Autodesk Inventor part; units mm, degrees
ref_plane "YZ Plane" through (0, 0, 0) normal (1, 0, 0) x (0, 1, 0)
ref_plane "XZ Plane" through (0, 0, 0) normal (0, 1, 0) x (-1, 0, 0)
ref_plane "XY Plane" through (0, 0, 0) normal (0, 0, 1) x (1, 0, 0)
sketch "Sketch1" plane through (0, 0, 0) normal (0, 1, 0) x (-1, 0, 0)
  line L0 (15, 25) -> (-15, 25)
  line L1 (-15, 25) -> (-15, -25)
  line L2 (-15, -25) -> (15, -25)
  line L3 (15, -25) -> (15, 25)
  line L4 (21, 0) -> (-21, 0) construction
  line L5 (0, -35) -> (0, 35) construction
  point P0 (0, 0)
  dimension "d11" = 15
  dimension "d12" = 15
  dimension "d13" = 25
  dimension "d14" = 25
extrude "Extrusion1" add sketch "Sketch1" against normal blind 1
fillet "Fillet1" radius 2.5 2 edges at (-15, -0.5, 25) (15, -0.5, 25)
fillet "Fillet2" radius 4 2 edges at (-15, -0.5, -25) (15, -0.5, -25)
sketch "Sketch3" plane through (0, 0, 0) normal (0, 1, 0) x (1, 0, 0)
  arc A0 (15, 21) -> (11, 25) centre (11, 21) ccw
  arc A1 (-11, 25) -> (-15, 21) centre (-11, 21) ccw
  line L0 (15, -22.5) -> (15, 21)
  line L1 (-15, 21) -> (-15, -22.5)
  line L2 (-12.5, -25) -> (12.5, -25)
  point P0 (0, 0)
  point P1 (11, -7)
  point P2 (-11, -8.5)
  point P3 (12.5, -25)
  dimension "d24" = 4
  dimension "d25" = 4
  dimension "d52" = 18
  dimension "d53" = 1.5
hole "Hole2" at (-11, 0, -21) at (11, 0, -21) at (11, 0, 7) at (-11, 0, 8.5) direction (0, -1, 0) diameter 3.4 end through all
properties part number "mcu_pcb"
The listing builds one solid part. Answer for the finished solid, in the listing's coordinates (mm). Give positions to 0.01 mm unless a question says otherwise; leave off trailing zeros. Write each loop counter-clockwise with the first axis right and the second up, starting at its lowest first coordinate (ties: lowest second). Pieces come first, ordered by that corner, then holes. Notation, with made-up numbers: (72.25, 63) -> (78.25, 63) arc R11 ccw to (78.25, 76) -> close; hole circle Ø1 at (42, 52.5). An arc over 180 degrees is marked (long way). One line per question, with ' | ' between items. Start each with the question number.
1. Section A-A (y = -0.25) is taken. Determine the outline of the cut face in (x, z), plus the area to 3 significant figures.
2. Find the intervals of material crossed by probe 1 along X at (y, z) = (-0.6, -21); probe 2 along Z at (x, y) = (11, -0.25); probe 3 along Z at (x, y) = (-9.75, -0.55), in increasing order.
3. For a pull along X with two mould halves and no side action, classify faces 1 (the cylindrical face through (-13.859, -0.507, -23.797)), 2 (the cylindrical face through (12.66, -0.51, 6.63)), 3 (the cylindrical face through (14.287, -0.507, 24.248)) as pulls with the +X half, pulls with the -X half, needs draft (parallel to the pull), parting line crosses it, or undercut.
Response values:
1) outline: (-15, -21) arc R4 ccw to (-11, -25) -> (11, -25) arc R4 ccw to (15, -21) -> (15, 22.5) arc R2.5 ccw to (12.5, 25) -> (-12.5, 25) arc R2.5 ccw to (-15, 22.5) -> close; hole circle Ø3.4 at (-11, -21); hole circle Ø3.4 at (-11, 8.5); hole circle Ø3.4 at (11, -21); hole circle Ø3.4 at (11, 7) | area: 1,450 mm2
2) probe 1: -15 to -12.7, -9.3 to 9.3, 12.7 to 15 | probe 2: -25 to -22.7, -19.3 to 5.3, 8.7 to 25 | probe 3: -25 to -22.15, -19.85 to 7.35, 9.65 to 25
3) face 1: pulls with the -X half | face 2: undercut | face 3: pulls with the +X half
